from build123d import *

# Parameters (mm, degrees)
BOSS_EXTRUDE1_DEPTH   = 14
SKETCH2_R             = 6
BOSS_EXTRUDE2_DEPTH   = 12
BOSS_EXTRUDE3_START   = 15
SKETCH3_R             = 6
BOSS_EXTRUDE3_DEPTH   = 15
BOSS_EXTRUDE4_DEPTH   = 10.5
M4_TAPPED_HOLE1_D     = 3.3
M4_TAPPED_HOLE1_DEPTH = 10.1
M4_TAPPED_HOLE1_TIP   = 0.991420021


with BuildPart() as part:
    # Sketch1 → Boss-Extrude1 (new body)
    with BuildSketch(Plane(origin=(0, 0, 0), x_dir=(1, 0, 0), z_dir=(0, 1, 0))):
        with BuildLine():
            Line((7.8, -2), (7.8, 2))
            Line((7.8, 2), (5.656854249, 2))
            ThreePointArc((5.656854249, 2), (-6, 0), (5.656854249, -2))
            Line((5.656854249, -2), (7.8, -2))
        make_face()
    extrude(amount=BOSS_EXTRUDE1_DEPTH)

    # Sketch2 → Boss-Extrude2 (add)
    with BuildSketch(Plane(origin=(0, 14, 0), x_dir=(1, 0, 0), z_dir=(0, 1, 0))):
        with Locations(Location((0, 0, 0), (0, 0, 19.471220634))):
            Circle(SKETCH2_R)
    extrude(amount=BOSS_EXTRUDE2_DEPTH)

    # Sketch3 → Boss-Extrude3 (add)
    with BuildSketch(Plane.XZ.offset(BOSS_EXTRUDE3_START)):
        with Locations(Location((0, 0, 0), (0, 0, 270))):
            Circle(SKETCH3_R)
    extrude(amount=-BOSS_EXTRUDE3_DEPTH)

    # Groove Sketch → Retaining Ring Groove (revolve, cut)
    with BuildSketch(Plane(origin=(1.604252923, 12.182890291, 0.373259529), x_dir=(-0.9343262431877186, 0.2824476966643587, -0.2173885230174828), z_dir=(-0.2266157025474993, 0, 0.9739842521103221)), mode=Mode.PRIVATE) as retaining_ring_groove_sk:
        with BuildLine():
            Line((10.535414006, -9.946396708), (11.998320123, -9.51566397))
            Line((11.998320123, -9.51566397), (11.800606735, -8.84416608))
            Line((11.800606735, -8.84416608), (10.337700618, -9.274898818))
            ThreePointArc((10.337700618, -9.274898818), (10.21858296, -9.371036434), (10.202333617, -9.523244897))
            Line((10.202333617, -9.523244897), (10.287067926, -9.811029707))
            ThreePointArc((10.287067926, -9.811029707), (10.383205542, -9.930147365), (10.535414006, -9.946396708))
        make_face()
    revolve(retaining_ring_groove_sk.sketch.rotate(Axis((0, 60.224615576, 0), (0, -1, 0)), 76.902094509), axis=Axis((0, 60.224615576, 0), (0, -1, 0)), mode=Mode.SUBTRACT)

    # Sketch5 → Boss-Extrude4 (add)
    with BuildSketch(Plane.XZ.offset(15)):
        Polygon((0, 5.773502692), (-5, 2.886751346), (-5, -2.886751346), (0, -5.773502692), (5, -2.886751346), (5, 2.886751346), align=None)
    extrude(amount=BOSS_EXTRUDE4_DEPTH)

    # M4 Tapped Hole1
    with Locations(Plane(origin=(0, -25.5, 0), x_dir=(-1, 0, 0), z_dir=(0, -1, 0))):
        with Locations((0, 0)):
            Hole(M4_TAPPED_HOLE1_D / 2, depth=M4_TAPPED_HOLE1_DEPTH)
            with Locations((0, 0, -(M4_TAPPED_HOLE1_DEPTH + M4_TAPPED_HOLE1_TIP / 2))):  # 118° drill point
                Cone(0, M4_TAPPED_HOLE1_D / 2, M4_TAPPED_HOLE1_TIP, mode=Mode.SUBTRACT)


solid = part.part
The listing builds one solid part. Answer for the finished solid, in the listing's coordinates (mm). A direction names the side the tool comes from. Coordinates: 2 decimals unless noted, no trailing zeros. Order: outer loops, then holes, each group sorted by start corner. A loop starts at its lowest first (then second) coordinate and runs counter-clockwise, first axis right, second up.
Q1. For a pull along X with two mould halves and no side action, classify faces 1 (the face through (5, -20, 0)), 2 (the face through (-1.216, -20.379, -1.115)), 3 (the face through (7, 0, 0)) as pulls with the +X half, pulls with the -X half, needs draft (parallel to the pull), parting line crosses it, or undercut.
Q2. Which of the six approach directions +Z, -Z, +X, -X, +Y, -Y give full straight-line access (tool end or side, diameter ignored) to faces 4 (the face through (-5.3, -15, 0)), 5 (the face through (-2.535, -20.176, -4.31)), 6 (the face through (7, 7, -2)), 7 (the face through (-3.32, 24.35, 4.32)), 8 (the face through (-5, -20, 0))?
Q3. A cutting plane is placed at B-B, the plane y = -10.5. Write down the section's boundary in (x, z).
Q4. Consider line 1 (Z direction, x = 0, y = -21.5); line 2 (Y direction, x = 0, z = 5.5); line 3 (Z direction, x = -1.25, y = -22.5). Determine where each line is inside the solid, lowest interval first.
Q5. Given P1, Ø1, axis at y = 18, z = 4, coming from the +X side; P2, Ø5, axis at x = -0.5, y = -13, coming from the +Z side; P3, Ø4.5, axis at y = -18, z = -1.5, coming from the +X side; P4, Ø1, axis at y = -18, z = 4.5, coming from the +X side, each flat-ended and moving along its own axis, determine where each tip first touches the part or whether it passes through.
Q6. A cutting plane is placed at A-A, the plane y = -20. Write down the section's boundary in (x, z).
Answers follow:
1. face 1: pulls with the +X half
1. face 2: undercut
1. face 3: needs draft
2. face 4: -Y
2. face 5: -Z, -X, -Y
2. face 6: -Z, +X, +Y, -Y
2. face 7: none
2. face 8: +Z, -Z, -X, -Y
3. outline: circle Ø12 at (0, 0)
4. line 1: z = -5.77 to -1.65, 1.65 to 5.77
4. line 2: y = -25.5 to 24.07, 24.63 to 26
4. line 3: z = -5.05 to -1.08, 1.08 to 5.05
5. P1: stops at x = 4.87
5. P2: stops at z = 6
5. P3: stops at x = 5
5. P4: stops at x = 3.07
6. outline: (-5, -2.89) - (0, -5.77) - (5, -2.89) - (5, 2.89) - (0, 5.77) - (-5, 2.89) - close; hole circle Ø3.3 at (0, 0)
